Here's the drawing with two shaded views (mm, measured from the low corner). I have some questions. A direction names the side the tool comes from. Give positions to 0.01 mm unless a question says otherwise; leave off trailing zeros. Write each loop counter-clockwise with the first axis right and the second up, starting at its lowest first coordinate (ties: lowest second). Pieces come first, ordered by that corner, then holes. Notation, with made-up numbers: (89.25, 49.25) -> (143.25, 49.25) arc R22 cw to (143.25, 78.25) -> close; hole circle Ø7 at (80, 49). An arc over 180 degrees is marked (long way). One line per question, with ' | ' between items.
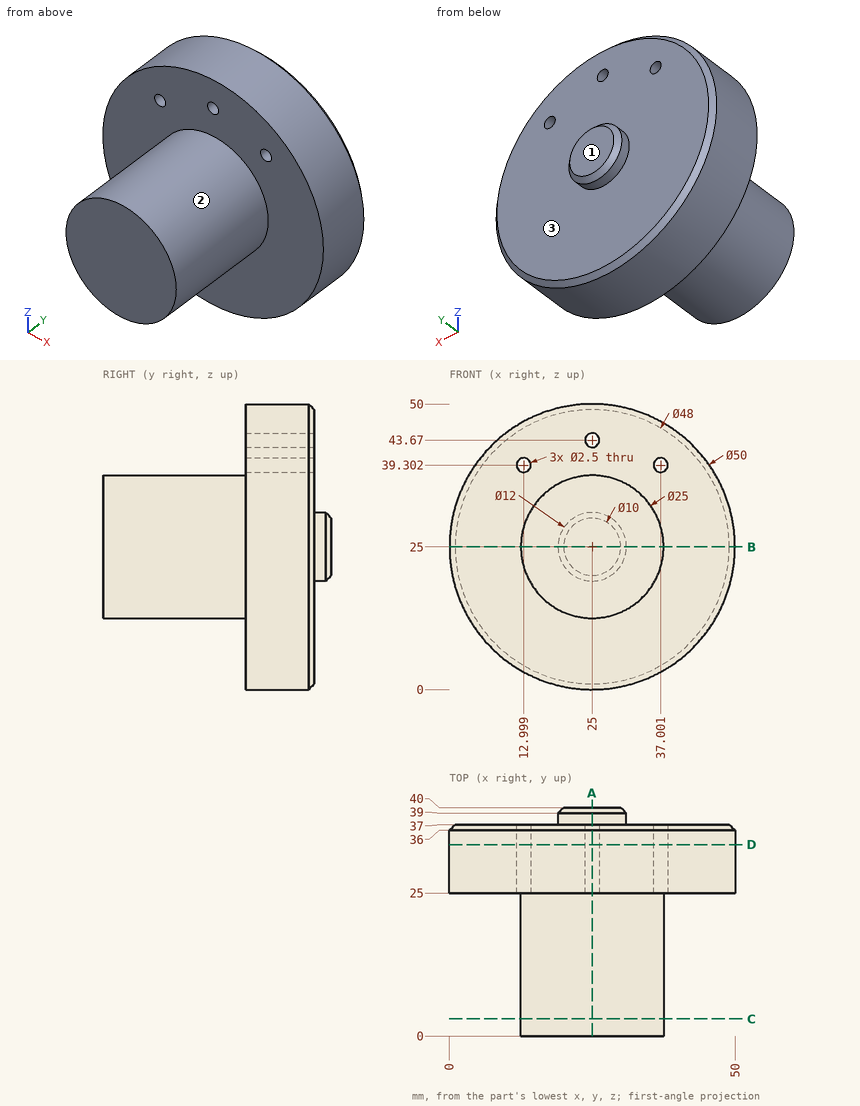
Q1. Imagine slicing it at A-A on x = 25. Please give me the cut outline in (y, z), and give its area (3 significant figures).
Answer below:
outline: (0, 12.5) -> (25, 12.5) -> (25, 0) -> (36, 0) -> (37, 1) -> (37, 19) -> (39, 19) -> (40, 20) -> (40, 30) -> (39, 31) -> (37, 31) -> (37, 42.42) -> (25, 42.42) -> (25, 37.5) -> (0, 37.5) -> close; (25, 44.92) -> (37, 44.92) -> (37, 49) -> (36, 50) -> (25, 50) -> close | area: 1,230 mm^2
Q2. Imagine slicing it at D-D on y = 33.5. Please give me the cut outline in (x, z).
Answer below:
outline: circle Ø50 at (25, 25); hole circle Ø2.5 at (13, 39.3); hole circle Ø2.5 at (25, 43.67); hole circle Ø2.5 at (37, 39.3)
Q3. On a 3-axis mill with a long thin cutter (end or side, diameter ignored), from which of +Z, -Z, +X, -X, +Y, -Y can I reach the whole of each face in a straight line? I mean the marked faces 1, 2 and 3. Say none if no direction works.
Answer below:
face 1: +Z, -Z, +X, -X, +Y | face 2: -Y | face 3: +Y
Q4. Imagine slicing it at C-C on y = 3. Please give me the cut outline in (x, z), and give its area (3 significant figures).
Answer below:
outline: circle Ø25 at (25, 25) | area: 491 mm^2
Q5. Will these pins go through, and if not, where does the flat tip stop? pin 1 (3 mm diameter, centred on y = 33.5, z = 39, fed in from -X); pin 2 (4 mm diameter, centred on x = 13.5, z = 37.5, fed in from -Y); pin 3 (8 mm diameter, centred on y = 5, z = 8, fed in from +X); pin 4 (1.5 mm diameter, centred on x = 14.5, y = 22.5, fed in from -Z).
Answer below:
pin 1: stops at x = 3.35 | pin 2: stops at y = 25 | pin 3: passes through | pin 4: stops at z = 17.18
Q6. If I drill on line 1 along Y through (x, z) = (16, 44); line 2 along X through (y, z) = (34, 25.5) (3 decimals); line 3 along Y through (x, z) = (16.5, 23.5), over which ranges is the centre line in solid material (lowest first)?
Answer below:
line 1: y = 25 to 37 | line 2: x = 0.005 to 49.995 | line 3: y = 0 to 37
Q7. Imagine slicing it at B-B on z = 25. Please give me the cut outline in (x, y).
Answer below:
outline: (0, 25) -> (12.5, 25) -> (12.5, 0) -> (37.5, 0) -> (37.5, 25) -> (50, 25) -> (50, 36) -> (49, 37) -> (31, 37) -> (31, 39) -> (30, 40) -> (20, 40) -> (19, 39) -> (19, 37) -> (1, 37) -> (0, 36) -> close
